Read the model definition and answer for the solid it produces. Units are mm, in the model's axes. A direction names the side the tool comes from. Coordinates: 2 decimals unless noted, no trailing zeros. Loops run counter-clockwise (first coordinate to the right, second up) from the corner with the lowest first, then second, coordinate; pieces in that order, holes last. Notation, with made-up numbers: (30, 5) -> (61, 5) arc R30 ccw to (61, 29) -> close; hole circle Ø5 at (73, 70). An arc over 180 degrees is marked (long way). Answer in a Markdown table with one row per item.
```python
from build123d import *

# Parameters (mm, degrees)
SKETCH_1_R          = 2.9
SKETCH_1_R_2        = 1.1
EXTRUDE_1_DEPTH     = 3
SKETCH_2_R          = 4.5
CUT_EXTRUDE_1_DEPTH = 1.5


with BuildPart() as part:
    # 草图1 → 凸台-拉伸1 (new body)
    with BuildSketch(Plane(origin=(0, 0, 0), x_dir=(1, 0, 0), z_dir=(0, 1, 0))):
        Polygon((-42, 47), (-42, 0), (-42, -47), (0, -47), (7, -47), (7, 47), (0, 47), align=None)
        with Locations((-35, -40)):
            Circle(SKETCH_1_R, mode=Mode.SUBTRACT)
        with Locations((-34, -30)):
            Circle(SKETCH_1_R_2, mode=Mode.SUBTRACT)
        Polygon((-35, -25), (-35, -4), (-21.05, -4), (-21.05, -40), (-25.5, -40), (-25.5, -25), align=None, mode=Mode.SUBTRACT)
        with Locations((0, -40)):
            Circle(SKETCH_1_R, mode=Mode.SUBTRACT)
        with Locations((-1.1, -30)):
            Circle(SKETCH_1_R_2, mode=Mode.SUBTRACT)
        Polygon((-1.1, -4), (-1.1, -25), (-10.6, -25), (-10.6, -40), (-15.05, -40), (-15.05, -4), align=None, mode=Mode.SUBTRACT)
        Polygon((-21.05, 4), (-35, 4), (-35, 25.5), (-25.5, 25.5), (-25.5, 40), (-21.05, 40), align=None, mode=Mode.SUBTRACT)
        with Locations((-34, 30)):
            Circle(SKETCH_1_R_2, mode=Mode.SUBTRACT)
        with Locations((-35, 40)):
            Circle(SKETCH_1_R, mode=Mode.SUBTRACT)
        Polygon((-10.6, 25.5), (-1.1, 25.5), (-1.1, 4), (-15.05, 4), (-15.05, 40), (-10.6, 40), align=None, mode=Mode.SUBTRACT)
        with Locations((-1.1, 30)):
            Circle(SKETCH_1_R_2, mode=Mode.SUBTRACT)
        with Locations((0, 40)):
            Circle(SKETCH_1_R, mode=Mode.SUBTRACT)
    extrude(amount=EXTRUDE_1_DEPTH)

    # 草图2 → 切除-拉伸1 (cut)
    with BuildSketch(Plane(origin=(0, 3, 0), x_dir=(1, 0, 0), z_dir=(0, 1, 0))):
        with Locations((-35, 40)):
            Circle(SKETCH_2_R)
        with Locations((0, 40)):
            Circle(SKETCH_2_R)
        with Locations((0, -40)):
            Circle(SKETCH_2_R)
        with Locations((-35, -40)):
            Circle(SKETCH_2_R)
    extrude(amount=-CUT_EXTRUDE_1_DEPTH, mode=Mode.SUBTRACT)


solid = part.part
```
1. A cutting plane is placed at A-A on z = -28. Give the vertices of the cut face in (x, y).
A:
| item | result |
|---|---|
| outline | (-42, 0) -> (-25.5, 0) -> (-25.5, 3) -> (-42, 3) -> close; (-21.05, 0) -> (-15.05, 0) -> (-15.05, 3) -> (-21.05, 3) -> close; (-10.6, 0) -> (7, 0) -> (7, 3) -> (-10.6, 3) -> close |
2. The mould has two halves that part along Z. Classify faces 1 (the flat face through (-35, 1, 15)), 2 (the flat face through (-17, 1, -47)), 3 (the flat face through (7, 1, 1)): pulls with the +Z half, pulls with the -Z half, needs draft (parallel to the pull), parting line crosses it, or undercut.
A:
| item | result |
|---|---|
| face 1 | undercut |
| face 2 | pulls with the -Z half |
| face 3 | needs draft |
3. Given pin 1 Ø2.5 at (x, z) = (-36, -39) entering from +Y; pin 2 Ø4.5 at (x, z) = (0.5, -41) entering from +Y, each flat-ended and moving along its own axis, determine where each tip first touches the part or whether it passes through.
A:
| item | result |
|---|---|
| pin 1 | passes through |
| pin 2 | stops at y = 1.5 |
4. A cutting plane is placed at C-C on y = 0.5. Count the separate pieces of the cut face and the enclosed holes in it, and give its area (3 significant figures).
A:
| item | result |
|---|---|
| separate pieces | 1 |
| enclosed holes | 12 |
| area | 3,040 mm2 |
5. Find the intervals of material crossed by probe 1 along X at (y, z) = (0.65, -15.5); probe 2 along Z at (x, y) = (-6, 2.3); probe 3 along Z at (x, y) = (-25, 2.75), in increasing order.
A:
| item | result |
|---|---|
| probe 1 | x = -42 to -35, -21.05 to -15.05, -1.1 to 7 |
| probe 2 | z = -47 to -25.5, -4 to 4, 25 to 47 |
| probe 3 | z = -47 to -40, -4 to 4, 40 to 47 |
6. A tool of negligible diameter and unlimited length cuts with its end or side. For faces 4 (the cylindrical face through (-32.92, 2.26, 43.99)), 5 (the flat face through (-18, 1, 47)), 6 (the flat face through (-10.6, 1, 32)), from which of +Z, -Z, +X, -X, +Y, -Y can it reach the whole face along a straight path? Write none if from no direction.
A:
| item | result |
|---|---|
| face 4 | +Y |
| face 5 | +Z, +X, -X, +Y, -Y |
| face 6 | +Y, -Y |
7. A cutting plane is placed at B-B on x = -8. Give the vertices of the cut face in (y, z), and give its area (4 significant figures).
A:
| item | result |
|---|---|
| outline | (0, -47) -> (3, -47) -> (3, -25.5) -> (0, -25.5) -> close; (0, -4) -> (3, -4) -> (3, 4) -> (0, 4) -> close; (0, 25) -> (3, 25) -> (3, 47) -> (0, 47) -> close |
| area | 154.5 mm2 |
